Could you check a few things on this drawing? It's one solid part, dimensions in mm from its lowest x, y, z. Give positions to 0.01 mm unless a question says otherwise; leave off trailing zeros. Loops run counter-clockwise (first coordinate to the right, second up) from the corner with the lowest first, then second, coordinate; pieces in that order, holes last.
Q1. Suppose I cut it at A-A (y = 9). List the corners of the cut face in (x, z) for me.
Q2. Suppose I cut it at C-C (z = 1.15). List the corners of the cut face in (x, y) for me.
Q3. Thinking about a two-plate mould opening in Y: for the marked faces 1, 2, 3 and 4, which applies, pulls with the +Y half, pulls with the -Y half, needs draft (parallel to the pull), parting line crosses it, or undercut?
Q4. Suppose I cut it at B-B (x = 45). List the corners of the cut face in (y, z) for me.
Q5. I'm going to push flat-ended pins straight in: P1, Ø3, axis at x = 18, y = 14.5, coming from the -Z side; P2, Ø9.5, axis at x = 45, y = 9, coming from the +Z side. Where does each tip first touch, or does it pass through?
Q6. I need wall thicknesses on probe 1 along X at (y, z) = (9, 2.25); probe 2 along Y at (x, z) = (10, 1.05); probe 3 along X at (y, z) = (11.5, 0.2). Which ranges of each line are inside material? Lowest first, please.
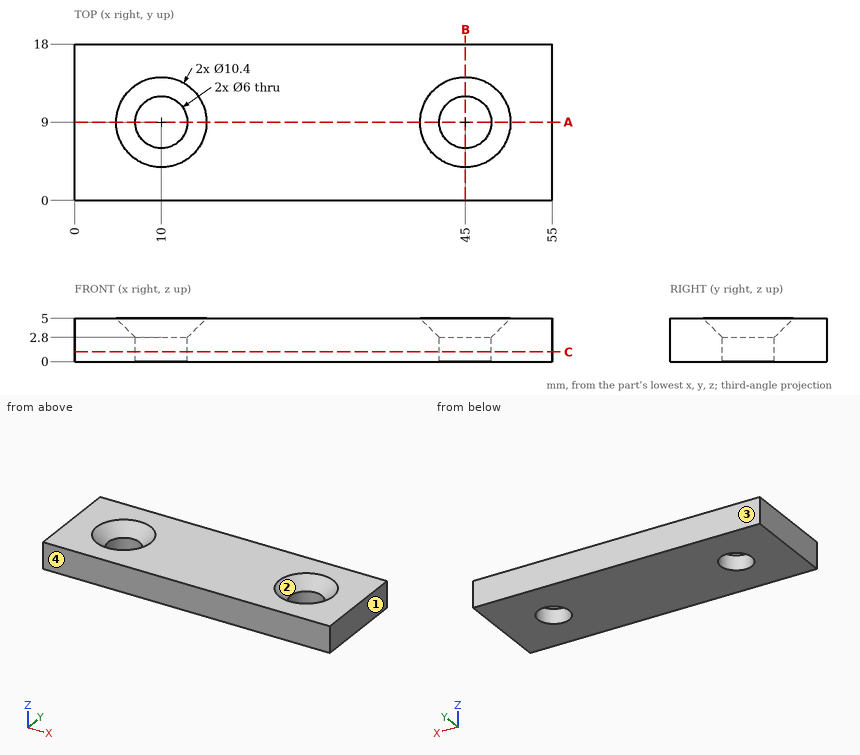
Solutions:
1. outline: (0, 0) - (7, 0) - (7, 2.8) - (4.8, 5) - (0, 5) - close; (13, 0) - (42, 0) - (42, 2.8) - (39.8, 5) - (15.2, 5) - (13, 2.8) - close; (48, 0) - (55, 0) - (55, 5) - (50.2, 5) - (48, 2.8) - close
2. outline: (0, 0) - (55, 0) - (55, 18) - (0, 18) - close; hole circle Ø6 at (10, 9); hole circle Ø6 at (45, 9)
3. face 1: needs draft
3. face 2: undercut
3. face 3: pulls with the +Y half
3. face 4: pulls with the -Y half
4. outline: (0, 0) - (6, 0) - (6, 2.8) - (3.8, 5) - (0, 5) - close; (12, 0) - (18, 0) - (18, 5) - (14.2, 5) - (12, 2.8) - close
5. P1: stops at z = 0
5. P2: stops at z = 4.55
6. probe 1: x = 0 to 7, 13 to 42, 48 to 55
6. probe 2: y = 0 to 6, 12 to 18
6. probe 3: x = 0 to 8.34, 11.66 to 43.34, 46.66 to 55
